The listing builds one solid part. Answer for the finished solid, in the listing's coordinates (mm). Face numbers are marked on the shaded views. A direction names the side the tool comes from. Coordinates: 2 decimals unless noted, no trailing zeros. Order: outer loops, then holes, each group sorted by start corner. A loop starts at its lowest first (then second) coordinate and runs counter-clockwise, first axis right, second up. Notation, with made-up numbers: (-32, 66.5) -> (-22, 66.5) arc R24 cw to (-22, 84.5) -> close; hole circle Ø2 at (38.25, 62.25). An arc over 180 degrees is marked (long way). Write item = value, one per line. Start each with the question number.
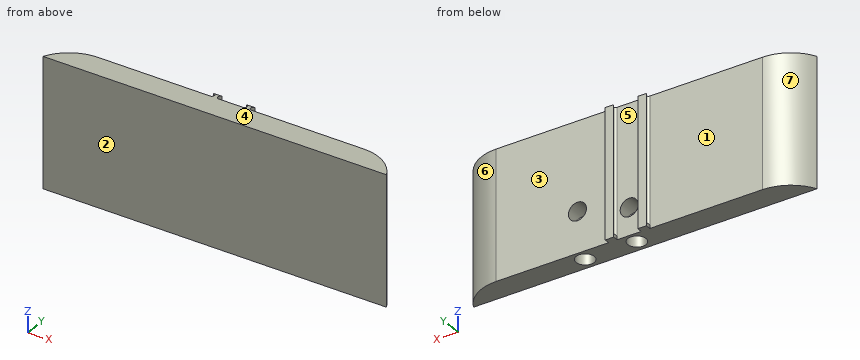
```python
from build123d import *

# Parameters (mm, degrees)
F0_R     = 5.25
F1_DEPTH = 75
F4_DEPTH = 2


# Not quite as in the source:
# - a feature names something its author has since deleted; it is built from what else it names


with BuildPart() as f1:
    # F0 (on Top) → F1 (new body)
    with BuildSketch(Plane.XY):
        with BuildLine():
            Line((-100, 0), (-13.8524602948, 0))
            Line((-13.8524602948, 0), (12.09906023, 0))
            Line((12.09906023, 0), (100, 0))
            ThreePointArc((100, 0), (90.75, 10.2142857143), (77.5, 14))
            Line((77.5, 14), (32.5911540906, 14))
            Line((32.5911540906, 14), (26.9999997473, 14))
            Line((26.9999997473, 14), (11.9999997473, 14))
            Line((11.9999997473, 14), (7, 14))
            Line((7, 14), (-7, 14))
            Line((-7, 14), (-11.9999997473, 14))
            Line((-11.9999997473, 14), (-77.5, 14))
            ThreePointArc((-77.5, 14), (-90.75, 10.2142857143), (-100, 0))
        make_face()
        with Locations((0, 7.25)):
            Circle(F0_R, mode=Mode.SUBTRACT)
        with Locations((30.1251118069, 7.25)):
            Circle(F0_R, mode=Mode.SUBTRACT)
        with Locations((30.1251118069, 7.25)):
            Circle(F0_R)
        with BuildLine():
            ThreePointArc((-11.9999997473, 17), (-10.4999997473, 15.5), (-11.9999997473, 14))
            Line((-11.9999997473, 14), (-7, 14))
            ThreePointArc((-7, 14), (-8.5, 15.5000001263), (-6.9999997473, 17))
            Line((-6.9999997473, 17), (-11.9999997473, 17))
        make_face()
        with BuildLine():
            ThreePointArc((6.9999998542, 17), (8.5, 15.5000000729), (7, 14))
            Line((7, 14), (11.9999997473, 14))
            ThreePointArc((11.9999997473, 14), (10.4999997473, 15.5), (11.9999997473, 17))
            Line((11.9999997473, 17), (6.9999998542, 17))
        make_face()
        with Locations((0, 7.25)):
            Circle(F0_R)
    extrude(amount=F1_DEPTH)

    # F0 (on Top) → F4 (join)
    with BuildSketch(Plane.XY):
        with BuildLine():
            ThreePointArc((11.9999997473, 17), (10.4999997473, 15.5), (11.9999997473, 14))
            Line((11.9999997473, 14), (11.9999997473, 17))
        make_face()
        with BuildLine():
            Line((6.9999998542, 17), (7, 14))
            ThreePointArc((7, 14), (8.5, 15.5000000729), (6.9999998542, 17))
        make_face()
        with BuildLine():
            ThreePointArc((-6.9999997473, 17), (-8.5, 15.5000001263), (-7, 14))
            Line((-7, 14), (-6.9999997473, 17))
        make_face()
        with BuildLine():
            Line((-11.9999997473, 17), (-11.9999997473, 14))
            ThreePointArc((-11.9999997473, 14), (-10.4999997473, 15.5), (-11.9999997473, 17))
        make_face()
        with BuildLine():
            ThreePointArc((-11.9999997473, 17), (-10.4999997473, 15.5), (-11.9999997473, 14))
            Line((-11.9999997473, 14), (-7, 14))
            ThreePointArc((-7, 14), (-8.5, 15.5000001263), (-6.9999997473, 17))
            Line((-6.9999997473, 17), (-11.9999997473, 17))
        make_face()
        with BuildLine():
            ThreePointArc((6.9999998542, 17), (8.5, 15.5000000729), (7, 14))
            Line((7, 14), (11.9999997473, 14))
            ThreePointArc((11.9999997473, 14), (10.4999997473, 15.5), (11.9999997473, 17))
            Line((11.9999997473, 17), (6.9999998542, 17))
        make_face()
    extrude(amount=F4_DEPTH)

    # F5: sweep along a path in F3
    with BuildLine(Plane.YZ.offset(30.1251118069)) as f5_path:
        Line((8, 0), (8, 23))
        Line((8, 23), (14, 23))
    # F0 (on Top) → F5 (sweep, cut)
    with BuildSketch(Plane.XY):
        with Locations((30.1251118069, 7.25)):
            Circle(F0_R)
    sweep(path=f5_path.line, transition=Transition.RIGHT, mode=Mode.SUBTRACT)

    # F7: sweep along a path in F6
    with BuildLine(Plane.YZ) as f7_path:
        Line((23.7799418298, 13.885), (9.2960403562, 13.885))
        Line((9.2960403562, 13.885), (9.2960403562, 0))
    # F0 (on Top) → F7 (sweep, cut)
    with BuildSketch(Plane.XY):
        with Locations((0, 7.25)):
            Circle(F0_R)
    sweep(path=f7_path.line, transition=Transition.RIGHT, mode=Mode.SUBTRACT)


solid = f1.part
```
Item 1: Section C-C, the plane y = 5 is taken. Give the vertices of the cut face in (x, z), then the cut area to 3 significant figures.
Item 2: Which of the six approach directions +Z, -Z, +X, -X, +Y, -Y give full straight-line access (tool end or side, diameter ignored) to the marked faces 1, 2 and 3?
Item 3: Section A-A, the plane x = 0 is taken. Give the vertices of the cut face in (y, z), then the cut area to 3 significant figures.
Item 4: Section B-B, the plane z = 43 is taken. Give the vertices of the cut face in (x, y), then the cut area to 3 significant figures.
Item 5: Each of these flat-tipped pins is pushed along its axis until it touches: pin 1 (0.8 mm diameter, centred on x = 7.5, y = 16, fed in from +Z); pin 2 (10 mm diameter, centred on y = 9.5, z = 54, fed in from -X); pin 3 (0.6 mm diameter, centred on y = 16, z = 1, fed in from +X). Where does it stop, or does it pass through?
Item 6: For a pull along X with two mould halves and no side action, classify the marked faces 4, 5, 6 and 7 as pulls with the +X half, pulls with the -X half, needs draft (parallel to the pull), parting line crosses it, or undercut.
Item 7: Section D-D, the plane x = 57.5 is taken. Give the vertices of the cut face in (y, z), then the cut area to 3 significant figures.
Item 8: Consider probe 1 along X at (y, z) = (15.75, 30); probe 2 along X at (y, z) = (4.5, 8); probe 3 along Y at (x, z) = (24, 61.5). Determine where each line is inside the solid, lowest interval first.
A:
q1.outline = (-96.75, 0) -> (-4.74, 0) -> (-4.74, 18.18) arc R5.25 cw to (4.74, 18.18) -> (4.74, 0) -> (25.38, 0) -> (25.38, 26) arc R5.25 cw to (34.87, 26) -> (34.87, 0) -> (96.75, 0) -> (96.75, 75) -> (-96.75, 75) -> close
q1.area = 14,100 mm^2
q2.face_1 = +Z, -Z, -X, +Y
q2.face_2 = +Z, -Z, +X, -X, -Y
q2.face_3 = +Z, -Z, +X, +Y
q3.outline = (0, 0) -> (2, 0) -> (2, 21.18) -> (14, 21.18) -> (14, 75) -> (0, 75) -> close; (12.5, 0) -> (14, 0) -> (14, 10.68) -> (12.5, 10.68) -> close
q3.area = 812 mm^2
q4.outline = (-100, 0) -> (100, 0) arc R25.08 ccw to (77.5, 14) -> (12, 14) arc R1.5 cw to (12, 17) -> (7, 17) arc R1.5 cw to (7, 14) -> (-7, 14) arc R1.5 cw to (-7, 17) -> (-12, 17) arc R1.5 cw to (-12, 14) -> (-77.5, 14) arc R25.08 ccw to start
q4.area = 2,640 mm^2
q5.pin_1 = 2
q5.pin_2 = -97.15
q5.pin_3 = 12
q6.face_4 = needs draft
q6.face_5 = undercut
q6.face_6 = pulls with the +X half
q6.face_7 = pulls with the -X half
q7.outline = (0, 0) -> (14, 0) -> (14, 75) -> (0, 75) -> close
q7.area = 1,050 mm^2
q8.probe_1 = -10.52 to -8.48, 8.48 to 10.52
q8.probe_2 = -97.15 to -4.47, 4.47 to 25.65, 34.6 to 97.15
q8.probe_3 = 0 to 14
